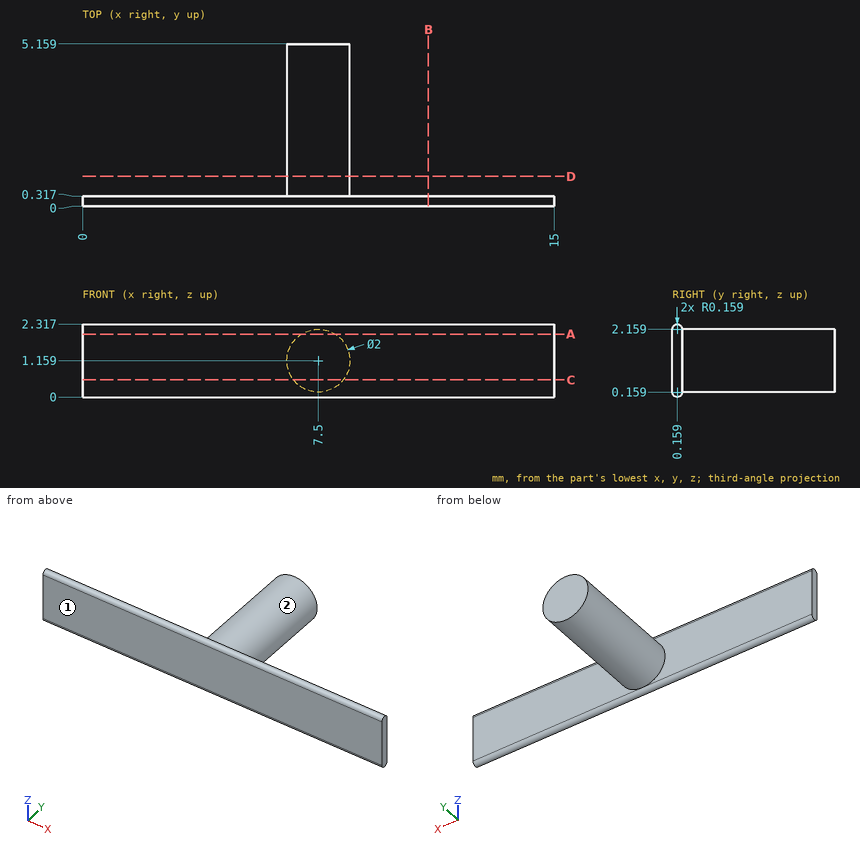
Geometry check sheet. Reference: drawing and pictorial views, mm from the part's lowest x, y, z. A direction names the side the tool comes from. Round coordinates to 2 decimals unless told otherwise and drop trailing zeros. Write each loop counter-clockwise with the first axis right and the second up, starting at its lowest first coordinate (ties: lowest second). Pieces come first, ordered by that corner, then holes. Notation, with made-up numbers: (23.5, 83) -> (67.5, 83) arc R18 cw to (67.5, 113) -> close; hole circle Ø8 at (-12, 84.25). An arc over 180 degrees is marked (long way). One line per question, with ' | ' between items. Start each with the question number.
1. Sectioned sample at D-D, the plane y = 0.95. Record the cut outline in (x, z).
2. Set-up check for the marked faces 1 and 2: record each of +Z, -Z, +X, -X, +Y, -Y from which the full face is reachable in a straight line by a thin tool's end or side.
3. Depth check by flat-ended pin: pin 1 (1 mm diameter, centred on y = 2.5, z = 1.5, fed in from -X); pin 2 (0.6 mm diameter, centred on x = 10, z = 1.5, fed in from +Y); pin 3 (1.5 mm diameter, centred on x = 8.5, y = 3.5, fed in from -Z). Enter the tip coordinate at first touch or a pass-through.
4. Sectioned sample at C-C, the plane z = 0.55. Record the cut outline in (x, y).
5. Sectioned sample at B-B, the plane x = 11. Record the cut outline in (y, z).
6. Scan lines: line 1 along Y through (x, z) = (1, 1.4); line 2 along Z through (x, y) = (7, 4.85) (1 decimal); line 3 along X through (y, z) = (3.8, 1.5). Record each from-to range of solid material in increasing order. Write a range as from..to.
7. Sectioned sample at A-A, the plane z = 2. Record the cut outline in (x, y).
Taken from the geometry:
1) outline: circle Ø2 at (7.5, 1.16)
2) face 1: +Z, -Z, +X, -X, -Y | face 2: +Y
3) pin 1: stops at x = 6.5 | pin 2: stops at y = 0.32 | pin 3: stops at z = 0.19
4) outline: (0, 0) -> (15, 0) -> (15, 0.32) -> (8.29, 0.32) -> (8.29, 5.16) -> (6.71, 5.16) -> (6.71, 0.32) -> (0, 0.32) -> close
5) outline: (0, 0.16) arc R0.16 ccw to (0.32, 0.16) -> (0.32, 2.16) arc R0.16 ccw to (0, 2.16) -> close
6) line 1: y = 0..0.32 | line 2: z = 0.3..2 | line 3: x = 6.56..8.44
7) outline: (0, 0) -> (15, 0) -> (15, 0.32) -> (8.04, 0.32) -> (8.04, 5.16) -> (6.96, 5.16) -> (6.96, 0.32) -> (0, 0.32) -> close
